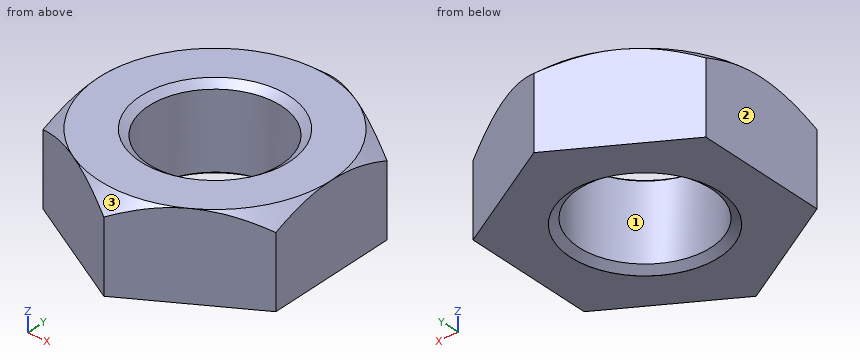
```python
from build123d import *

# Parameters (mm, degrees)
THREADSCHEMATIC_START     = -29.6926
THREADSCHEMATIC_OUTLINE_R = 22.62124
THREADSCHEMATIC_DEPTH     = 29.6926


# Read off the part's stored shape, not the designer's step: ThreadSchematic
with BuildPart() as part:
    # ThreadSchematic outline → ThreadSchematic (new body)
    with BuildSketch(Plane.XY.offset(THREADSCHEMATIC_START)):
        Polygon((39.6875, 22.913588808), (0, 45.827177617), (-39.6875, 22.913588808), (-39.6875, -22.913588808), (0, -45.827177617), (39.6875, -22.913588808), align=None)
        Circle(THREADSCHEMATIC_OUTLINE_R, mode=Mode.SUBTRACT)
    extrude(amount=THREADSCHEMATIC_DEPTH)

    # Sketch2 → Single-Chamfer (revolve, cut)
    with BuildSketch(Plane(origin=(0, 0, 0), x_dir=(0, 0, -1), z_dir=(1, 0, 0))):
        Polygon((0, 39.6875), (-12.7, 39.6875), (-12.7, 58.527177617), (5.08, 58.527177617), (5.08, 45.827177617), align=None)
    revolve(axis=Axis((0, 0, 0), (0, 0, -1)), mode=Mode.SUBTRACT)

    # Sketch3 → EndChamfer (revolve, cut)
    with BuildSketch(Plane(origin=(0, 0, 0), x_dir=(0, 0, -1), z_dir=(1, 0, 0)), mode=Mode.PRIVATE) as endchamfer_sk:
        Polygon((29.6672, 25.4), (27.526920431, 22.343364), (29.718, 22.343364), (29.718, 25.4), align=None)
        Polygon((-0.0508, 25.4), (0, 25.4), (2.140279569, 22.343364), (-0.0508, 22.343364), align=None)
    revolve(endchamfer_sk.sketch.rotate(Axis((0, 0, -25.037505729), (0, 0, -1)), 90), axis=Axis((0, 0, -25.037505729), (0, 0, -1)), mode=Mode.SUBTRACT)


solid = part.part
```
Part model, mm, in its own coordinate system. Face numbers are marked on the shaded views. Coordinates: 2 decimals unless noted, no trailing zeros. Order: outer loops, then holes, each group sorted by start corner. A loop starts at its lowest first (then second) coordinate and runs counter-clockwise, first axis right, second up. Notation, with made-up numbers: (58.5, 8.5) - (81.5, 8.5) arc R20 ccw to (81.5, 40.5) - close; hole circle Ø5 at (56, 84). An arc over 180 degrees is marked (long way). Return JSON: item names as keys, results as strings. Group by question number.
Item 1: Cut at A-A (z = -7). List the corners of the cut face in (x, y), plus the area to 3 significant figures.
Item 2: Drill centre lines: probe 1 along Y at (x, z) = (0, -11); probe 2 along X at (y, z) = (-1, -22.25); probe 3 along X at (y, z) = (15.5, -24.5). Where is each one in solid material? Low to high. Write a range as from..to.
Item 3: Pull direction X, two halves, no side cores. Call the marked faces 1, 2 and 3: pulls with the +X half, pulls with the -X half, needs draft (parallel to the pull), parting line crosses it, or undercut.
Item 4: Pin check, flat tips, straight feed: pin 1 (2 mm diameter, centred on x = 25.5, z = -12.5, fed in from +Y); pin 2 (12 mm diameter, centred on y = 25.5, z = -7.5, fed in from -X); pin 3 (6 mm diameter, centred on x = 20, y = -9.5, fed in from -Z); pin 4 (2 mm diameter, centred on x = -13, z = -26.5, fed in from +Y). Stop position of each tip, or through.
Check values:
{
 "1": {"outline": "(-39.69, -22.91) - (0, -45.83) - (39.69, -22.91) - (39.69, 22.91) - (0, 45.83) - (-39.69, 22.91) - close; hole circle Ø45.24 at (0, 0)", "area": "3,850 mm2"},
 "2": {"probe 1": "y = -45.83..-22.62, 22.62..45.83", "probe 2": "x = -39.69..-22.6, 22.6..39.69", "probe 3": "x = -39.69..-16.48, 16.48..39.69"},
 "3": {"face 1": "undercut", "face 2": "pulls with the -X half", "face 3": "parting line crosses it"},
 "4": {"pin 1": "stops at y = 31.68", "pin 2": "stops at x = -39.69", "pin 3": "stops at z = -29.49", "pin 4": "stops at y = 38.9"}
}
